Could you check a few things on this model? Use its own coordinates, in mm. Face numbers are marked on the shaded views. Round coordinates to 2 decimals unless told otherwise and drop trailing zeros. Loops run counter-clockwise (first coordinate to the right, second up) from the corner with the lowest first, then second, coordinate; pieces in that order, holes last. Notation, with made-up numbers: (72, 41) -> (82, 41) arc R23 ccw to (82, 78) -> close; hole circle Ø6 at (73, -2). An arc over 180 degrees is marked (long way). One line per item, written item: value.
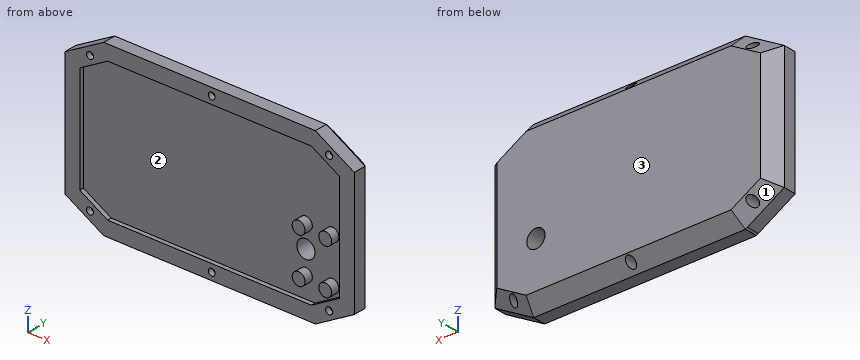
Autodesk Inventor part; units mm, degrees
ref_plane "YZ Plane" through (0, 0, 0) normal (1, 0, 0) x (0, 1, 0)
ref_plane "XZ Plane" through (0, 0, 0) normal (0, 1, 0) x (-1, 0, 0)
ref_plane "XY Plane" through (0, 0, 0) normal (0, 0, 1) x (1, 0, 0)
sketch "Sketch5" plane through (0, 0, 0) normal (0, 1, 0) x (-1, 0, 0)
  line L0 (0, 0) -> (-95, 0)
  line L1 (-95, 0) -> (-95, -65)
  line L2 (-95, -65) -> (0, -65)
  line L3 (0, -65) -> (0, 0)
  line L4 (0, -65) -> (12.9904, -57.5)
  line L5 (12.9904, -57.5) -> (12.9904, -7.5)
  line L6 (12.9904, -7.5) -> (0, 0)
  line L7 (-95, -65) -> (-107.9904, -57.5)
  line L8 (-107.9904, -57.5) -> (-107.9904, -7.5)
  line L9 (-107.9904, -7.5) -> (-95, 0)
  dimension "d23" = 95
  dimension "d24" = 65
  dimension "d25" = 15
  dimension "d26" = 15
  dimension "d27" = 120
  dimension "d28" = 15
  dimension "d29" = 15
  dimension "d30" = 120
extrude "Extrusion3" add sketch "Sketch5" along normal blind 10
sketch "Sketch6" plane through (0, 0, 0) normal (0, -1, 0) x (1, 0, 0)
  line L0 (0, 7) -> (87, 7)
  line L1 (95, -72) -> (8, -72)
  line L2 (0, 0) -> (95, 0)
  line L3 (95, -65) -> (0, -65)
  line L4 (96.8756, 7) -> (114.9904, -3.4585)
  line L5 (95, 0) -> (107.9904, -7.5)
  line L6 (114.9904, -3.4585) -> (114.9904, -61.5415)
  line L7 (107.9904, -7.5) -> (107.9904, -57.5)
  line L8 (96.8756, -72) -> (114.9904, -61.5415)
  line L9 (107.9904, -57.5) -> (95, -65)
  line L10 (107.9904, -57.5) -> (95, -65)
  line L11 (87, 7) -> (96.8756, 7)
  line L12 (95, -72) -> (96.8756, -72)
  line L13 (0, 7) -> (-1.8756, 7)
  line L14 (-19.9904, -3.4585) -> (-1.8756, 7)
  line L15 (-19.9904, -61.5415) -> (-2.8038, -71.4641)
  line L16 (0, -65) -> (-12.9904, -57.5)
  line L17 (-12.9904, -7.5) -> (0, 0)
  line L18 (-19.9904, -61.5415) -> (-19.9904, -3.4585)
  line L19 (-12.9904, -57.5) -> (-12.9904, -7.5)
  line L20 (0, -65) -> (-12.9904, -57.5)
  line L21 (-12.9904, -7.5) -> (-12.9904, -57.5)
  line L22 (-12.9904, -57.5) -> (0, -65)
  line L23 (95, -65) -> (0, -65)
  line L24 (0, -65) -> (95, -65)
  line L25 (95, -65) -> (107.9904, -57.5)
  line L26 (107.9904, -7.5) -> (107.9904, -57.5)
  line L27 (95, 0) -> (107.9904, -7.5)
  line L28 (107.9904, -7.5) -> (95, 0)
  line L29 (0, 0) -> (-12.9904, -7.5)
  line L30 (95, 0) -> (0, 0)
  line L31 (8, -72) -> (-1.8756, -72)
  line L32 (-2.8038, -71.4641) -> (-1.8756, -72)
  dimension "d33" = 7
  dimension "d34" = 7
  dimension "d35" = 7
  dimension "d36" = 7
  dimension "d37" = 7
  dimension "d38" = 7
  dimension "d39" = 7
  dimension "d40" = 7
extrude "Extrusion4" add sketch "Sketch6" along normal blind 2 and the other way blind 10
chamfer "Chamfer1" distance 6 angle 45 8 edges at (47.5, 10, 7) (-10.933, 10, 1.7707) (-19.9904, 10, -32.5) (-10.933, 10, -66.7707) (47.5, 10, -72) (105.933, 10, -66.7707) (114.9904, 10, -32.5) (105.933, 10, 1.7707)
sketch "Sketch7" plane through (0, 0, 0) normal (0, -1, 0) x (1, 0, 0)
  line L0 (86.4904, -40.25) -> (94.9904, -40.25)
  line L1 (94.9904, -40.25) -> (94.9904, -48.75)
  line L2 (94.9904, -48.75) -> (86.4904, -48.75)
  line L3 (86.4904, -48.75) -> (86.4904, -40.25)
  line L4 (96.8756, 7) -> (-1.8756, 7)
  line L5 (114.9904, -61.5415) -> (114.9904, -3.4585)
  circle A0 centre (90.7404, -55) radius 3
  circle A1 centre (90.7404, -34) radius 3
  circle A2 centre (103.1404, -34) radius 3
  circle A3 centre (103.1404, -55) radius 3
  circle A4 centre (90.7404, -44.5) radius 4.25
  circle A5 centre (46.5, 2.8174) radius 1.834
  circle A6 centre (46.5, -64.297) radius 1.834
  line L6 (-1.8756, -72) -> (96.8756, -72)
  point P0 (0, 0)
  dimension "d48" = 8.5
  dimension "d50" = 20
  dimension "d51" = 6.25
  dimension "d52" = 8.15
  dimension "d53" = 12.4
  dimension "d54" = 0
  dimension "d55" = 21
  dimension "d56" = 12.4
  dimension "d57" = 0
  dimension "d58" = 0
  dimension "d59" = 6
  dimension "d61" = 8.5
  dimension "d107" = 27.5
sketch "Sketch9" plane through (0, -2, 0) normal (0, -1, 0) x (1, 0, 0)
  circle A0 centre (-8.2452, -0.7189) radius 1.6
  line L0 (0, -65) -> (-12.9904, -57.5)
  line L1 (0, -65) -> (-1.8756, -72)
  line L2 (95, -65) -> (0, -65)
  line L3 (107.9904, -7.5) -> (107.9904, -57.5)
  line L4 (0, 0) -> (95, 0)
  line L5 (-12.9904, -7.5) -> (-16.4904, -1.4378)
  line L6 (-19.9904, -3.4585) -> (-1.8756, 7)
  line L7 (0, 0) -> (-3.5, 6.0622)
  line L8 (-12.9904, -57.5) -> (-19.9904, -61.5415)
  line L9 (-12.9904, -57.5) -> (-15.4904, -61.8301)
  line L10 (0, -65) -> (-2.5, -69.3301)
  line L11 (95, -65) -> (97.5, -69.3301)
  line L12 (95, 0) -> (98.5, 6.0622)
  line L13 (96.8756, 7) -> (114.9904, -3.4585)
  line L14 (107.9904, -7.5) -> (114.9904, -3.4585)
  line L15 (107.9904, -7.5) -> (111.4904, -1.4378)
  line L16 (107.9904, -57.5) -> (111.4904, -63.5622)
  line L17 (96.8756, -72) -> (114.9904, -61.5415)
  line L18 (107.9904, -57.5) -> (95, -65)
  line L19 (95, 0) -> (107.9904, -7.5)
  circle A1 centre (-8.2452, -64.2811) radius 1.6
  circle A2 centre (103.2452, -64.2811) radius 1.6
  circle A3 centre (103.2452, -0.7189) radius 1.6
  circle A4 centre (48.5, 3.5) radius 1.6
  circle A5 centre (48.5, -68.5) radius 1.6
  line L20 (95, -65) -> (95, -72)
  line L21 (-1.8756, -72) -> (96.8756, -72)
  line L22 (95, 0) -> (95, 7)
  line L23 (96.8756, 7) -> (-1.8756, 7)
  dimension "d62" = 90
  dimension "d63" = 90
  dimension "d64" = 90
  dimension "d65" = 7.5
  dimension "d66" = 3.5
  dimension "d67" = 3.2
  dimension "d68" = 7.5
  dimension "d69" = 3.5
  dimension "d70" = 3.5
  dimension "d71" = 7.5
  dimension "d72" = 7.5
  dimension "d73" = 3.5
  dimension "d76" = 3.5
  dimension "d77" = 46.5
  dimension "d78" = 3.5
  dimension "d79" = 46.5
extrude "Extrusion6" cut sketch "Sketch9" against normal blind 2.5 contours A0 | A1 | A2 | A3 | A4 | A5
sketch "Sketch13" plane through (48.5, 0.5, 3.5) normal (0, -1, 0) x (1, 0, 0)
  circle A0 centre (0, 0) radius 2
  circle A1 centre (54.7452, -4.2189) radius 2
  circle A2 centre (54.7452, -67.7811) radius 2
  circle A3 centre (0, -72) radius 2
  circle A4 centre (-56.7452, -67.7811) radius 2
  circle A5 centre (-56.7452, -4.2189) radius 2
  circle A6 centre (-56.7452, -4.2189) radius 1.6
  circle A7 centre (0, 0) radius 1.6
  circle A8 centre (54.7452, -4.2189) radius 1.6
  circle A9 centre (54.7452, -67.7811) radius 1.6
  circle A10 centre (0, -72) radius 1.6
  circle A11 centre (-56.7452, -67.7811) radius 1.6
  point P0 (-48.5, -3.5)
  dimension "d90" = 4
  dimension "d91" = 4
  dimension "d92" = 4
  dimension "d93" = 4
  dimension "d94" = 4
  dimension "d95" = 4
extrude "Extrusion7" cut sketch "Sketch13" against normal blind 10 contours A0 | A1 | A2 | A3 | A4 | A5 | A6 | A7 | A8 | A9 | A10 | A11
extrude "Extrusion8" add sketch "Sketch7" along normal blind 4 contours A0 | A1 | A2 | A3
sketch "Sketch14" plane through (0, 0, 0) normal (0, -1, 0) x (1, 0, 0)
  line L0 (86.4904, -48.75) -> (94.9904, -48.75)
  line L1 (94.9904, -48.75) -> (94.9904, -40.25)
  line L2 (94.9904, -40.25) -> (86.4904, -40.25)
  line L3 (86.4904, -40.25) -> (86.4904, -48.75)
  line L4 (95, -65) -> (0, -65)
  line L5 (107.9904, -7.5) -> (107.9904, -57.5)
  circle A0 centre (90.7404, -44.5) radius 4.25
  circle A1 centre (90.7404, -55) radius 3
  point P0 (0, 0)
  dimension "d100" = 8.5
  dimension "d101" = 8.5
  dimension "d103" = 13
  dimension "d104" = 8.5
  dimension "d108" = 9.25
extrude "Extrusion9" cut sketch "Sketch14" against normal blind 10 contours A0
properties part number "Topv3"
Item 1: If we mould it in two halves opening along Z, with no side actions, what happens to the marked faces 1, 2 and 3? For each: released by +Z, released by -Z, zero draft, split by the parting line, or undercut.
Output:
face 1: released by -Z
face 2: undercut
face 3: zero draft
Item 2: If we section it at D-D on z = 3.5: List the corners of the cut face in (x, y) for me, plus the area to 3 significant figures.
Output:
outline: (-7.94, -2) -> (46.9, -2) -> (46.9, 0.5) -> (46.5, 0.5) -> (46.5, 7.5) -> (-0.94, 7.5) -> (-7.94, 4) -> close; (50.1, -2) -> (102.94, -2) -> (102.94, 4) -> (95.94, 7.5) -> (50.5, 7.5) -> (50.5, 0.5) -> (50.1, 0.5) -> close
area: 993 mm²
Item 3: I need wall thicknesses on line 1 (Z direction, x = 48.5, y = -0.6); line 2 (Z direction, x = 48.5, y = 2.75); line 3 (Z direction, x = 48.5, y = 4.25). Which ranges of each line are inside material? Lowest first, please. Write a range as from..to.
Output:
line 1: z = -72..-70.1, -66.9..-65, 0..1.9, 5.1..7
line 2: z = -72..-70.5, -66.5..1.5, 5.5..7
line 3: z = -71.75..-70.5, -66.5..1.5, 5.5..6.75
Item 4: If we section it at A-A on x = 48.5: List the corners of the cut face in (y, z) for me, plus the area to 3 significant figures.
Output:
outline: (-2, -72) -> (4, -72) -> (5.5, -70.5) -> (0.5, -70.5) -> (0.5, -70.1) -> (-2, -70.1) -> close; (-2, -66.9) -> (0.5, -66.9) -> (0.5, -66.5) -> (9.5, -66.5) -> (10, -66) -> (10, 1) -> (9.5, 1.5) -> (0.5, 1.5) -> (0.5, 1.9) -> (-2, 1.9) -> (-2, 0) -> (0, 0) -> (0, -65) -> (-2, -65) -> close; (-2, 5.1) -> (0.5, 5.1) -> (0.5, 5.5) -> (5.5, 5.5) -> (4, 7) -> (-2, 7) -> close
area: 710 mm²
Item 5: If we section it at B-B on z = -44.5: List the corners of the cut face in (x, y) for me.
Output:
outline: (-19.99, -2) -> (-12.99, -2) -> (-12.99, 0) -> (86.49, 0) -> (86.49, 10) -> (-13.99, 10) -> (-19.99, 4) -> close; (94.99, 0) -> (107.99, 0) -> (107.99, -2) -> (114.99, -2) -> (114.99, 4) -> (108.99, 10) -> (94.99, 10) -> close
Item 6: Will these pins go through, and if not, where does the flat tip stop? pin 1 Ø3 at (x, z) = (47.5, -68.5) entering from +Y; pin 2 Ø13.5 at (x, z) = (90.74, -44.5) entering from +Y; pin 3 Ø3.5 at (x, z) = (103.25, -0.72) entering from +Y; pin 4 Ø1.5 at (y, z) = (6, -10) entering from -X.
Output:
pin 1: stops at y = 8.95
pin 2: stops at y = 10
pin 3: stops at y = 0.5
pin 4: stops at x = -18.74
Item 7: If we section it at C-C on z = -26: List the corners of the cut face in (x, y) for me.
Output:
outline: (-19.99, -2) -> (-12.99, -2) -> (-12.99, 0) -> (107.99, 0) -> (107.99, -2) -> (114.99, -2) -> (114.99, 4) -> (108.99, 10) -> (-13.99, 10) -> (-19.99, 4) -> close
